Here's how the part is built. I have some questions about the finished solid (model axes, mm). Face numbers are marked on the shaded views. A direction names the side the tool comes from. Round coordinates to 2 decimals unless told otherwise and drop trailing zeros. Order: outer loops, then holes, each group sorted by start corner. A loop starts at its lowest first (then second) coordinate and runs counter-clockwise, first axis right, second up. Notation, with made-up numbers: (13, 79) - (31, 79) arc R32 cw to (31, 113) - close; hole circle Ø3 at (30.25, 32). An arc over 180 degrees is marked (long way). Answer as a JSON object with one key per item and string values.
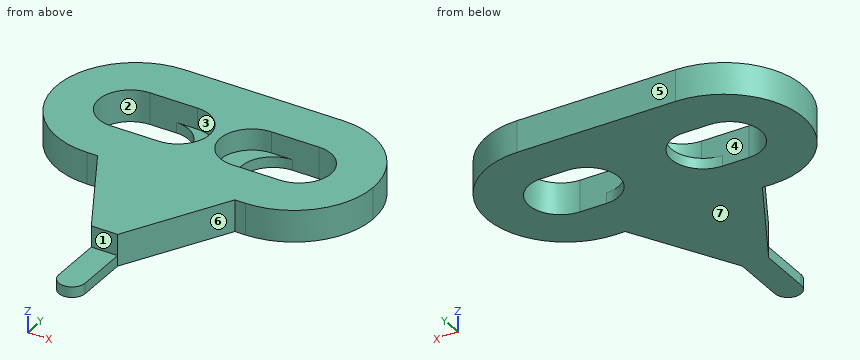
```python
from build123d import *

# Parameters (mm, degrees)
PAD_DEPTH    = 1
PAD001_DEPTH = 2


with BuildPart() as part:
    # Sketch → Pad (new body)
    with BuildSketch(Plane.XY):
        with BuildLine():
            ThreePointArc((-7.5, 7.5), (-15, 0), (-7.5, -7.5))
            Line((-7.5, -7.5), (-6.5, -7.5))
            Line((-1.25, -17), (-6.5, -7.5))
            Line((-1.25, -22), (-1.25, -17))
            ThreePointArc((-1.25, -22), (0, -23.25), (1.25, -22))
            Line((1.25, -22), (1.25, -17))
            Line((1.25, -17), (6.5, -7.5))
            Line((6.5, -7.5), (7.5, -7.5))
            ThreePointArc((7.5, -7.5), (12.803301, -5.303301), (15, 0))
            ThreePointArc((15, 0), (12.803311, 5.303291), (7.500028, 7.5))
            Line((-7.5, 7.5), (7.500028, 7.5))
        make_face()
        with BuildLine():
            ThreePointArc((-8, 3), (-11, 0), (-8, -3))
            Line((-8, -3), (-5.5, -3))
            ThreePointArc((-5.5, -3), (-2.5, 0), (-5.5, 3))
            Line((-8, 3), (-5.5, 3))
        make_face(mode=Mode.SUBTRACT)
        with BuildLine():
            ThreePointArc((5.5, 3), (2.5, 0), (5.5, -3))
            Line((5.5, -3), (8, -3))
            ThreePointArc((8, -3), (11, 0), (8, 3))
            Line((5.5, 3), (8, 3))
        make_face(mode=Mode.SUBTRACT)
    extrude(amount=PAD_DEPTH)

    # Sketch001 (on Face21 of Pad) → Pad001 (join)
    with BuildSketch(Plane.XY.offset(1)):
        with BuildLine():
            ThreePointArc((-7.5, 7.5), (-15, 0), (-7.5, -7.5))
            Line((-7.5, -7.5), (-6.5, -7.5))
            Line((-1.25, -17), (-6.5, -7.5))
            Line((-1.25, -17), (1.25, -17))
            Line((1.25, -17), (6.5, -7.5))
            Line((6.5, -7.5), (7.5, -7.5))
            ThreePointArc((7.5, -7.5), (12.803301, -5.303301), (15, 0))
            ThreePointArc((15, 0), (12.803291, 5.303311), (7.499972, 7.5))
            Line((-7.5, 7.5), (7.499972, 7.5))
        make_face()
        with BuildLine():
            ThreePointArc((-8, 3), (-11, 0), (-8, -3))
            Line((-8, -3), (-3.5, -3))
            ThreePointArc((-3.5, -3), (-0.5, 0), (-3.5, 3))
            Line((-8, 3), (-3.5, 3))
        make_face(mode=Mode.SUBTRACT)
        with BuildLine():
            ThreePointArc((3.5, 3), (0.5, 0), (3.5, -3))
            Line((3.5, -3), (8, -3))
            ThreePointArc((8, -3), (11, 0), (8, 3))
            Line((3.5, 3), (8, 3))
        make_face(mode=Mode.SUBTRACT)
    extrude(amount=PAD001_DEPTH)


solid = part.part
```
1. For P1, Ø0.9, axis at x = 6, z = 1, coming from the -Y side; P2, Ø1, axis at x = -0.5, z = 2, coming from the -Y side; P3, Ø6, axis at x = 11.5, y = -10.5, coming from the +Z side; P4, Ø1.1, axis at y = -18.5, z = 0.5, coming from the -X side, each with a flat end and sliding along its axis, tell me the tip position at first contact or that it passes through.
Responses:
{"P1": "y = -9.22", "P2": "y = -17", "P3": "through", "P4": "x = -1.25"}
2. Thinking about a two-plate mould opening in Y: for the marked faces 4, 5, 6 and 7, which applies, pulls with the +Y half, pulls with the -Y half, needs draft (parallel to the pull), parting line crosses it, or undercut?
Responses:
{"face 4": "undercut", "face 5": "pulls with the +Y half", "face 6": "pulls with the -Y half", "face 7": "needs draft"}
3. Imagine slicing it at C-C (x = -3). List the corners of the cut face in (y, z) for me, plus the area to 3 significant figures.
Responses:
{"outline": "(-13.83, 0) - (-1.66, 0) - (-1.66, 1) - (-2.96, 1) - (-2.96, 3) - (-13.83, 3) - close; (1.66, 0) - (7.5, 0) - (7.5, 3) - (2.96, 3) - (2.96, 1) - (1.66, 1) - close", "area": "48.9 mm2"}
4. For the marked faces 1, 2 and 3, which set-ups out of +Z, -Z, +X, -X, +Y, -Y let a thin tool reach every point of the face, with its end or its side?
Responses:
{"face 1": "+Z, +X, -X, -Y", "face 2": "+Z, -Z", "face 3": "+Z"}
5. If I drill on L1, parallel to X at y = 0, z = 1.95; L2, parallel to Y at x = 7.5, z = 2.85; L3, parallel to X at y = 1, z = 1.45, over which ranges is the centre line in solid material (lowest first)? Write a range as [from, to].
Responses:
{"L1": "[-15, -11], [-0.5, 0.5], [11, 15]", "L2": "[-7.5, -3], [3, 7.5]", "L3": "[-14.93, -10.83], [-0.67, 0.67], [10.83, 14.93]"}
6. Imagine slicing it at D-D (z = 0.55). List the corners of the cut face in (x, y) for me, plus the area to 3 significant figures.
Responses:
{"outline": "(-7.5, -7.5) - (-6.5, -7.5) - (-1.25, -17) - (-1.25, -22) arc R1.25 ccw to (1.25, -22) - (1.25, -17) - (6.5, -7.5) - (7.5, -7.5) arc R7.5 ccw to (7.5, 7.5) - (-7.5, 7.5) arc R7.5 ccw to start; hole (-8, -3) - (-5.5, -3) arc R3 ccw to (-5.5, 3) - (-8, 3) arc R3 ccw to start; hole (5.5, -3) - (8, -3) arc R3 ccw to (8, 3) - (5.5, 3) arc R3 ccw to start", "area": "404 mm2"}
7. Imagine slicing it at A-A (z = 2.45). List the corners of the cut face in (x, y) for me.
Responses:
{"outline": "(-7.5, -7.5) - (-6.5, -7.5) - (-1.25, -17) - (1.25, -17) - (6.5, -7.5) - (7.5, -7.5) arc R7.5 ccw to (7.5, 7.5) - (-7.5, 7.5) arc R7.5 ccw to start; hole (-8, -3) - (-3.5, -3) arc R3 ccw to (-3.5, 3) - (-8, 3) arc R3 ccw to start; hole (3.5, -3) - (8, -3) arc R3 ccw to (8, 3) - (3.5, 3) arc R3 ccw to start"}
8. Imagine slicing it at B-B (y = -0.5). List the corners of the cut face in (x, z) for me.
Responses:
{"outline": "(-14.98, 0) - (-10.96, 0) - (-10.96, 3) - (-14.98, 3) - close; (-2.54, 0) - (2.54, 0) - (2.54, 1) - (0.54, 1) - (0.54, 3) - (-0.54, 3) - (-0.54, 1) - (-2.54, 1) - close; (10.96, 0) - (14.98, 0) - (14.98, 3) - (10.96, 3) - close"}
